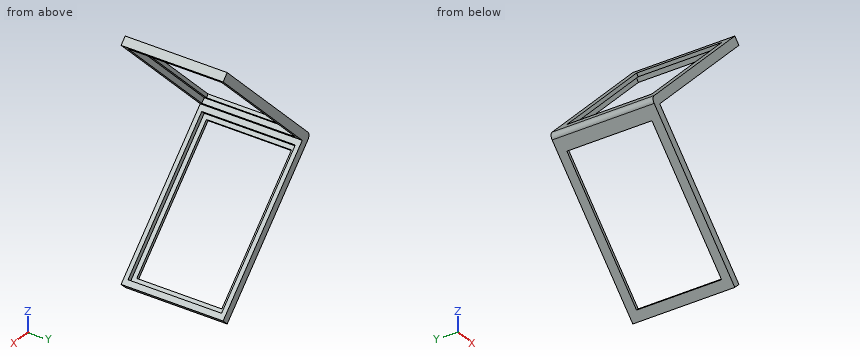
Autodesk Inventor part; units mm, degrees
ref_plane "YZ Plane" through (0, 0, 0) normal (1, 0, 0) x (0, 1, 0)
ref_plane "XZ Plane" through (0, 0, 0) normal (0, 1, 0) x (-1, 0, 0)
ref_plane "XY Plane" through (0, 0, 0) normal (0, 0, 1) x (1, 0, 0)
sketch "Sketch4" plane through (0, 0, 0) normal (0, 1, 0) x (-1, 0, 0)
  line L0 (0, 0) -> (-71.842, 71.842)
  line L1 (0, 0) -> (101.6, 0) construction
  line L2 (0, 0) -> (-71.842, -71.842)
  line L3 (0, 0) -> (101.6, 0) construction
  line L4 (-71.842, 71.842) -> (-75.3776, 68.3065)
  line L5 (-75.3776, 68.3065) -> (-7.0711, 0)
  line L6 (-7.0711, 0) -> (-75.3776, -68.3065)
  line L7 (-75.3776, -68.3065) -> (-71.842, -71.842)
  dimension "d20" = 101.6
  dimension "d21" = 135
  dimension "d22" = 101.6
  dimension "d23" = 135
  dimension "d24" = 5
extrude "Extrusion3" add sketch "Sketch4" along normal blind 60
sketch "Sketch5" plane through (7.0711, 0, 0) normal (0.7071, 0, -0.7071) x (-0.7071, 0, -0.7071)
  line L0 (-96.6, 0) -> (0, 0)
  line L1 (0, 0) -> (0, 60)
  line L2 (-96.6, 60) -> (0, 60)
  line L3 (-96.6, 0) -> (-96.6, 60)
  line L4 (-96.6, 0) -> (0, 0)
  line L5 (-96.6, 60) -> (0, 0)
  line L6 (0, 0) -> (-96.6, 0)
  line L7 (0, 60) -> (5, 60)
  line L8 (-96.6, 0) -> (0, 60)
  line L9 (-93.3, 2.5) -> (-3.3, 2.5)
  line L10 (-3.3, 2.5) -> (-3.3, 57.5)
  line L11 (-3.3, 57.5) -> (-93.3, 57.5)
  line L12 (-93.3, 57.5) -> (-93.3, 2.5)
  line L13 (-93.3, 2.5) -> (-3.3, 57.5) construction
  line L14 (-3.3, 2.5) -> (-93.3, 57.5) construction
  point P0 (5, 0)
  point P1 (-48.3, 30)
  dimension "d27" = 90
  dimension "d28" = 55
extrude "Extrusion4" cut sketch "Sketch5" against normal blind 3 contours L9 L12 L11 L5 L8 | L8 L5 L9 | L5 L8 L11 L10 L9 | L11 L8 L5
sketch "Sketch6" plane through (4.9497, 0, 2.1213) normal (0.7071, 0, -0.7071) x (-0.7071, 0, -0.7071)
  line L0 (-93.3, 2.5) -> (-93.3, 57.5)
  line L1 (-3.3, 2.5) -> (-93.3, 2.5)
  line L2 (-3.3, 57.5) -> (-3.3, 2.5)
  line L3 (-93.3, 57.5) -> (-3.3, 57.5)
  line L4 (-90.8, 5) -> (-5.8, 5)
  line L5 (-5.8, 5) -> (-5.8, 55)
  line L6 (-5.8, 55) -> (-90.8, 55)
  line L7 (-90.8, 55) -> (-90.8, 5)
  line L8 (-90.8, 5) -> (-5.8, 55) construction
  line L9 (-5.8, 5) -> (-90.8, 55) construction
  point P0 (5, 0)
  point P1 (-48.3, 30)
  dimension "d31" = 85
  dimension "d32" = 50
extrude "Extrusion5" cut sketch "Sketch6" against normal blind 3 contours L7 L6 L5 L4
sketch "Sketch7" plane through (75.3776, 0, -68.3065) normal (0.7071, 0, 0.7071) x (0.7071, 0, -0.7071)
  line L0 (-96.6, 0) -> (0, 0)
  line L1 (0, 0) -> (0, 60)
  line L2 (-96.6, 60) -> (0, 60)
  line L3 (-96.6, 0) -> (-96.6, 60)
  line L4 (-96.6, 0) -> (0, 60)
  line L5 (-96.6, 60) -> (0, 0)
  line L6 (-93.3, 2.5) -> (-3.3, 2.5)
  line L7 (-3.3, 2.5) -> (-3.3, 57.5)
  line L8 (-3.3, 57.5) -> (-93.3, 57.5)
  line L9 (-93.3, 57.5) -> (-93.3, 2.5)
  line L10 (-93.3, 2.5) -> (-3.3, 57.5) construction
  line L11 (-3.3, 2.5) -> (-93.3, 57.5) construction
  point P0 (-101.6, 0)
  point P1 (-48.3, 30)
  dimension "d35" = 90
  dimension "d36" = 55
extrude "Extrusion6" cut sketch "Sketch7" against normal blind 3 contours L6 L9 L8 L5 L4 | L4 L5 L6 | L5 L4 L8 L7 L6 | L8 L4 L5
sketch "Sketch8" plane through (73.2563, 0, -70.4278) normal (0.7071, 0, 0.7071) x (0.7071, 0, -0.7071)
  line L0 (-93.3, 2.5) -> (-93.3, 57.5)
  line L1 (-3.3, 2.5) -> (-93.3, 2.5)
  line L2 (-3.3, 57.5) -> (-3.3, 2.5)
  line L3 (-93.3, 57.5) -> (-3.3, 57.5)
  line L4 (-90.8, 5) -> (-5.8, 5)
  line L5 (-5.8, 5) -> (-5.8, 55)
  line L6 (-5.8, 55) -> (-90.8, 55)
  line L7 (-90.8, 55) -> (-90.8, 5)
  line L8 (-90.8, 5) -> (-5.8, 55) construction
  line L9 (-5.8, 5) -> (-90.8, 55) construction
  point P0 (-101.6, 0)
  point P1 (-48.3, 30)
  dimension "d39" = 85
  dimension "d40" = 50
extrude "Extrusion7" cut sketch "Sketch8" against normal blind 3 contours L7 L6 L5 L4
fillet "Fillet1" radius 3.175 1 edges at (0, 30, 0)
properties part number "SolarPannelMounting"
Build history of the part. All positions in model axes, mm. Round coordinates to 2 decimals unless told otherwise and drop trailing zeros. Loops run counter-clockwise (first coordinate to the right, second up) from the corner with the lowest first, then second, coordinate; pieces in that order, holes last.
Item 1: Drill centre lines: line 1 along Y through (x, z) = (30, 28.5); line 2 along Z through (x, y) = (25.5, 56.5); line 3 along X through (y, z) = (13, -2). Where is each one in solid material? Low to high.
Item 2: Saw through at A-A (y = 18.5). State how many separate pieces and enclosed holes the cut face has, then the cut area to 3 significant figures.
Item 3: Saw through at B-B (z = -17). List the corners of the cut face in (x, y), then the cut area to 3 significant figures.
Item 4: Saw through at C-C (x = 45). List the corners of the cut face in (y, z).
Item 5: Pin check, flat tip, straight feed: P1, Ø5, axis at x = 9.5, y = 29, coming from the +Z side. Stop position of the tip, or through.
Worked answers:
1. line 1: y = 0 to 5, 55 to 60
1. line 2: z = -25.5 to -22.67, 22.67 to 25.5
1. line 3: x = 2.02 to 9.07
2. separate pieces: 3
2. enclosed holes: 0
2. area: 109 mm2
3. outline: (17, 0) - (24.07, 0) - (24.07, 2.5) - (19.83, 2.5) - (19.83, 5) - (17, 5) - close; (17, 55) - (19.83, 55) - (19.83, 57.5) - (24.07, 57.5) - (24.07, 60) - (17, 60) - close
3. area: 49.5 mm2
4. outline: (0, -45) - (5, -45) - (5, -42.17) - (2.5, -42.17) - (2.5, -37.93) - (0, -37.93) - close; (0, 37.93) - (2.5, 37.93) - (2.5, 42.17) - (5, 42.17) - (5, 45) - (0, 45) - close; (55, -45) - (60, -45) - (60, -37.93) - (57.5, -37.93) - (57.5, -42.17) - (55, -42.17) - close; (55, 42.17) - (57.5, 42.17) - (57.5, 37.93) - (60, 37.93) - (60, 45) - (55, 45) - close
5. P1: stops at z = 7.64
